Work out the finished part from the listing and answer in its coordinate system (mm). Face numbers are marked on the shaded views. Round coordinates to 2 decimals unless told otherwise and drop trailing zeros. Write each loop counter-clockwise with the first axis right and the second up, starting at its lowest first coordinate (ties: lowest second). Pieces come first, ordered by that corner, then holes. Notation, with made-up numbers: M 71.25,-4 L 125.25,-4 A22 ccw 125.25,2 Z; hole C 47,-9.5 d10. An arc over 180 degrees is marked long. One line per item, written item: value. Start each with the question number.
Q1. Consider probe 1 along Y at (x, z) = (0, 15); probe 2 along Y at (x, z) = (0, 6); probe 3 along Y at (x, z) = (3, 21.5). Determine where each line is inside the solid, lowest interval first.
Q2. The mould has two halves that part along Y. Classify the marked faces 1, 2, 3 and 4: released by +Y, released by -Y, zero draft, split by the parting line, or undercut.
Q3. Find section A-A (x = 0). Write down the section's boundary in (y, z), and give its area (3 significant figures).
Q4. Given pin 1 Ø4 at (x, z) = (7.5, 19.5) entering from +Y; pin 2 Ø13 at (x, y) = (-34.64, -20) entering from -Z; pin 3 Ø8 at (x, y) = (9, 40) entering from +Z; pin 4 Ø1 at (y, z) = (53.5, 4.5) entering from +X, each flat-ended and moving along its own axis, determine where each tip first touches the part or whether it passes through.
Q5. Find section C-C (y = -20). Write down the section's boundary in (x, z), and give its area (3 significant figures).
Q6. Find section D-D (z = 18.5). Write down the section's boundary in (x, y).
Q7. Find section B-B (x = -7). Write down the section's boundary in (y, z), and give its area (3 significant figures).
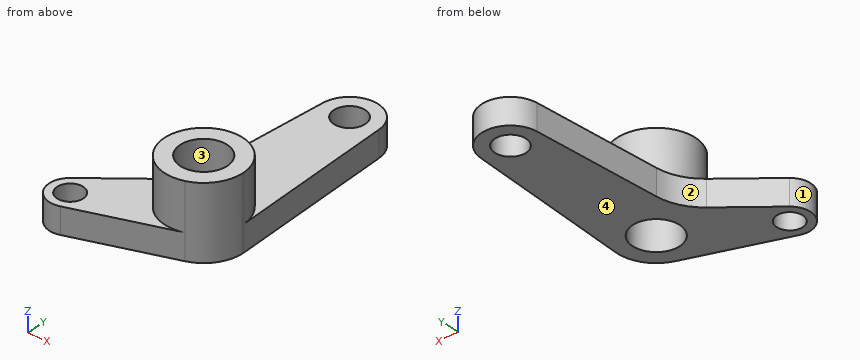
from build123d import *

# Parameters (mm, degrees)
F0_R     = 9
F1_DEPTH = 28
F0_R_2   = 5
F0_R_3   = 6
F2_DEPTH = 10


with BuildPart() as f1:
    # F0 (on Top) → F1 (new body)
    with BuildSketch(Plane.XY):
        with BuildLine():
            ThreePointArc((5.110947, -14.102419), (12.281372, -8.612079), (15, 0))
            ThreePointArc((15, 0), (14.992891, 0.461757), (14.971571, 0.923077))
            ThreePointArc((14.971571, 0.923077), (-12.540664, 8.22993), (5.110947, -14.102419))
        make_face()
        Circle(F0_R, mode=Mode.SUBTRACT)
    extrude(amount=F1_DEPTH)

    # F0 (on Top) → F2 (join)
    with BuildSketch(Plane.XY):
        with BuildLine():
            ThreePointArc((5.110947, -14.102419), (12.281372, -8.612079), (15, 0))
            ThreePointArc((15, 0), (14.992891, 0.461757), (14.971571, 0.923077))
            ThreePointArc((14.971571, 0.923077), (-12.540664, 8.22993), (5.110947, -14.102419))
        make_face()
        Circle(F0_R, mode=Mode.SUBTRACT)
        with BuildLine():
            ThreePointArc((5.110947, -14.102419), (-12.540664, 8.22993), (14.971571, 0.923077))
            Line((14.971571, 0.923077), (10.979152, 65.676923))
            ThreePointArc((10.979152, 65.676923), (0, 76), (-10.979152, 65.676923))
            Line((-10.979152, 65.676923), (-14.048582, 15.893218))
            ThreePointArc((-14.048582, 15.893218), (-16.147129, 8.129895), (-21.133903, 1.820762))
            Line((-21.133903, 1.820762), (-39.791725, -13.87871))
            ThreePointArc((-39.791725, -13.87871), (-41.569219, -24), (-31.915178, -27.52129))
            Line((-31.915178, -27.52129), (5.110947, -14.102419))
        make_face()
        with Locations((-34.641016, -20)):
            Circle(F0_R_2, mode=Mode.SUBTRACT)
        with Locations((0, 65)):
            Circle(F0_R_3, mode=Mode.SUBTRACT)
    extrude(amount=F2_DEPTH)


solid = f1.part
The answers:
1. probe 1: -15 to -9, 9 to 15
1. probe 2: -15.95 to -9, 9 to 59, 71 to 76
1. probe 3: -14.7 to -8.49, 8.49 to 14.7
2. face 1: split by the parting line
2. face 2: released by +Y
2. face 3: undercut
2. face 4: zero draft
3. outline: M -15.95,0 L -9,0 L -9,28 L -15,28 L -15,10 L -15.95,10 Z; M 9,0 L 59,0 L 59,10 L 15,10 L 15,28 L 9,28 Z; M 71,0 L 76,0 L 76,10 L 71,10 Z
3. area: 836 mm2
4. pin 1: y = 13.96
4. pin 2: z = 0
4. pin 3: z = 10
4. pin 4: x = 11.76
5. outline: M -42.64,0 L -39.64,0 L -39.64,10 L -42.64,10 Z; M -29.64,0 L -11.16,0 L -11.16,10 L -29.64,10 Z
5. area: 215 mm2
6. outline: M 14.97,0.92 A15 ccw long 15,0 A15 ccw Z; hole C 0,0 d18
7. outline: M -18.49,0 L -5.66,0 L -5.66,28 L -13.27,28 L -13.27,10 L -18.49,10 Z; M 5.66,0 L 73.49,0 L 73.49,10 L 13.27,10 L 13.27,28 L 5.66,28 Z
7. area: 1,080 mm2
